from build123d import *

# Parameters (mm, degrees)
SKETCH_1_R      = 22
SKETCH_1_R_2    = 3.1
SKETCH_1_R_3    = 1.6
EXTRUDE_1_DEPTH = 2
SKETCH_3_R      = 11
SKETCH_3_R_2    = 7.6
EXTRUDE_2_DEPTH = 5
SKETCH_2_R      = 7
SKETCH_2_R_2    = 5.1
EXTRUDE_3_DEPTH = 6


with BuildPart() as part:
    # 草图1 → 凸台-拉伸1 (new body)
    with BuildSketch(Plane.XY):
        Circle(SKETCH_1_R)
        Circle(SKETCH_1_R_2, mode=Mode.SUBTRACT)
        with Locations((0, 16)):
            Circle(SKETCH_1_R_3, mode=Mode.SUBTRACT)
        with Locations((15.216904261, 4.94427191)):
            Circle(SKETCH_1_R_3, mode=Mode.SUBTRACT)
        with Locations((9.404564037, -12.94427191)):
            Circle(SKETCH_1_R_3, mode=Mode.SUBTRACT)
        with Locations((-9.404564037, -12.94427191)):
            Circle(SKETCH_1_R_3, mode=Mode.SUBTRACT)
        with Locations((-15.216904261, 4.94427191)):
            Circle(SKETCH_1_R_3, mode=Mode.SUBTRACT)
    extrude(amount=EXTRUDE_1_DEPTH)

    # 草图3 → 凸台-拉伸2 (add)
    with BuildSketch(Plane(origin=(0, 0, 0), x_dir=(-1, 0, 0), z_dir=(0, 0, -1))):
        with Locations(Location((0, 0, 0), (0, 0, 180))):
            Circle(SKETCH_3_R)
        Circle(SKETCH_3_R_2, mode=Mode.SUBTRACT)
    extrude(amount=EXTRUDE_2_DEPTH)

    # 草图2 → 凸台-拉伸3 (add)
    with BuildSketch(Plane.XY.offset(2)):
        Circle(SKETCH_2_R)
        Circle(SKETCH_2_R_2, mode=Mode.SUBTRACT)
    extrude(amount=EXTRUDE_3_DEPTH)


solid = part.part
The listing builds one solid part. Answer for the finished solid, in the listing's coordinates (mm). A direction names the side the tool comes from. Coordinates: 2 decimals unless noted, no trailing zeros. Order: outer loops, then holes, each group sorted by start corner. A loop starts at its lowest first (then second) coordinate and runs counter-clockwise, first axis right, second up. Notation, with made-up numbers: (-17.75, 45) -> (-12.75, 45) arc R23 cw to (-12.75, 77) -> close; hole circle Ø2 at (66.5, 85.25). An arc over 180 degrees is marked (long way). Answer in a Markdown table with one row per item. Add a question column.
Item 1: Find section D-D (z = 0.75). Write down the section's boundary in (x, y), then the cut area to 3 significant figures.
Item 2: Find section A-A (x = 0). Write down the section's boundary in (y, z), then the cut area to 3 significant figures.
Item 3: Find section B-B (y = 0). Write down the section's boundary in (x, z).
Item 4: Each of these flat-tipped pins is pushed along its axis until it touches: P1, Ø2, axis at x = -2.5, y = 11, coming from the -Z side; P2, Ø7.5, axis at x = 0.5, y = -1, coming from the -Z side; P3, Ø9, axis at x = 0, y = 0, coming from the +Z side; P4, Ø6, axis at y = 6.5, z = 6, coming from the -X side. Where does it stop, or does it pass through?
Item 5: Find the intervals of material crossed by L1, parallel to Y at x = 0, z = -3.9; L2, parallel to Y at x = 0, z = 3.75; L3, parallel to Z at x = -5.5, y = 19, in increasing order. Write a range as from..to.
Item 6: Find section C-C (x = -15). Write down the section's boundary in (y, z).
Item 7: Which of the six approach directions +Z, -Z, +X, -X, +Y, -Y give full straight-line access (tool end or side, diameter ignored) to faces 4 (the face through (16.08, 6.29, 0.99)), 5 (the face through (3.3, 0.1, 0)), 6 (the face through (-5.2, 5.2, 2))?
Item 8: Determine the mould class of faces 1 (the face through (5, 10, 0)), 2 (the face through (-11.003, -12.874, 0.986)), 3 (the face through (6.466, -2.681, 4.958)) for opening direction Y: +Y half, -Y half, draft (parallel to the pull), parting line (faces both ways), or undercut.
Result set:
| question | item | result |
|---|---|---|
| 1 | outline | circle Ø44 at (0, 0); hole circle Ø3.2 at (-15.22, 4.94); hole circle Ø3.2 at (-9.4, -12.94); hole circle Ø6.2 at (0, 0); hole circle Ø3.2 at (0, 16); hole circle Ø3.2 at (9.4, -12.94); hole circle Ø3.2 at (15.22, 4.94) |
| 1 | area | 1,450 mm² |
| 2 | outline | (-22, 0) -> (-11, 0) -> (-11, -5) -> (-7.6, -5) -> (-7.6, 0) -> (-3.1, 0) -> (-3.1, 2) -> (-5.1, 2) -> (-5.1, 8) -> (-7, 8) -> (-7, 2) -> (-22, 2) -> close; (3.1, 0) -> (7.6, 0) -> (7.6, -5) -> (11, -5) -> (11, 0) -> (14.4, 0) -> (14.4, 2) -> (7, 2) -> (7, 8) -> (5.1, 8) -> (5.1, 2) -> (3.1, 2) -> close; (17.6, 0) -> (22, 0) -> (22, 2) -> (17.6, 2) -> close |
| 2 | area | 126 mm² |
| 3 | outline | (-22, 0) -> (-11, 0) -> (-11, -5) -> (-7.6, -5) -> (-7.6, 0) -> (-3.1, 0) -> (-3.1, 2) -> (-5.1, 2) -> (-5.1, 8) -> (-7, 8) -> (-7, 2) -> (-22, 2) -> close; (3.1, 0) -> (7.6, 0) -> (7.6, -5) -> (11, -5) -> (11, 0) -> (22, 0) -> (22, 2) -> (7, 2) -> (7, 8) -> (5.1, 8) -> (5.1, 2) -> (3.1, 2) -> close |
| 4 | P1 | stops at z = -5 |
| 4 | P2 | stops at z = 0 |
| 4 | P3 | stops at z = 2 |
| 4 | P4 | stops at x = -6.06 |
| 5 | L1 | y = -11..-7.6, 7.6..11 |
| 5 | L2 | y = -7..-5.1, 5.1..7 |
| 5 | L3 | z = 0..2 |
| 6 | outline | (-16.09, 0) -> (3.36, 0) -> (3.36, 2) -> (-16.09, 2) -> close; (6.53, 0) -> (16.09, 0) -> (16.09, 2) -> (6.53, 2) -> close |
| 7 | face 4 | +Z, -Z |
| 7 | face 5 | -Z |
| 7 | face 6 | +Z |
| 8 | face 1 | draft |
| 8 | face 2 | undercut |
| 8 | face 3 | parting line |
